The listing builds one solid part. Answer for the finished solid, in the listing's coordinates (mm). Coordinates: 2 decimals unless noted, no trailing zeros. Loops run counter-clockwise (first coordinate to the right, second up) from the corner with the lowest first, then second, coordinate; pieces in that order, holes last. Notation, with made-up numbers: M 45,67 L 97,67 A17 cw 97,80 Z; hole C -1,77 d4. An arc over 180 degrees is marked long. Return JSON: item names as keys, results as strings. Group by question number.
1. Section C-C (y = 0.8) is taken. Write down the section's boundary in (x, z) (3 decimals).
2. Given P1, Ø3, axis at x = 7.5, z = -37.5, coming from the -Y side; P2, Ø1, axis at y = 1, z = -23.5, coming from the +X side; P3, Ø1, axis at x = 12.5, y = 1.5, coming from the +Z side; P4, Ø1.6, axis at y = 2.5, z = 4.5, coming from the +X side, each flat-ended and moving along its own axis, determine where each tip first touches the part or whether it passes through.
3. Section B-B (x = 22.5) is taken. Write down the section's boundary in (y, z) (3 decimals), then the cut area to 3 significant figures.
4. Section D-D (x = 7) is taken. Write down the section's boundary in (y, z) (3 decimals).
5. Straight lines are drawn through the part: L1, parallel to X at y = 1.9, z = -5; L2, parallel to Z at x = 36, y = 1.8; L3, parallel to X at y = 1.55, z = 3.5. For each, find the intervals that lie inside material, in ascending order. Write a range as from..to.
6. Section A-A (z = -5) is taken. Write down the section's boundary in (x, y) (3 decimals).
```python
from build123d import *

# Parameters (mm, degrees)
SKETCH1_R           = 1.27
BOSS_EXTRUDE1_DEPTH = 3.175
FILLET1_R           = 2.921
SKETCH5_W           = 22
SKETCH5_H           = 3.175
BOSS_EXTRUDE3_DEPTH = 3.175
SKETCH2_W           = 6
SKETCH2_H           = 3.175
BOSS_EXTRUDE2_DEPTH = 3.175


with BuildPart() as part:
    # Sketch1 → Boss-Extrude1 (new body)
    with BuildSketch(Plane(origin=(0, 0, 0), x_dir=(1, 0, 0), z_dir=(0, 1, 0))):
        Polygon((0, 0), (0, 47.63), (10, 47.63), (39.73, 10), (39.73, 0), align=None)
        with Locations(Location((3.683, 43.74, 0), (0, 0, 270))):
            Circle(SKETCH1_R, mode=Mode.SUBTRACT)
        with Locations(Location((36.043, 5, 0), (0, 0, 270))):
            Circle(SKETCH1_R, mode=Mode.SUBTRACT)
        Polygon((10, 35.531824847), (10, 10), (30.171702171, 10), align=None, mode=Mode.SUBTRACT)
    extrude(amount=BOSS_EXTRUDE1_DEPTH)

    # Fillet1
    fillet1_edges = [part.edges().sort_by_distance(p)[0] for p in [
        (10, 1.5875, -10),
        (30.171702171, 1.5875, -10),
        (10, 1.5875, -35.531824847),
        (0, 1.5875, 0),
        (0, 1.5875, -47.63),
        (10, 1.5875, -47.63),
        (39.73, 1.5875, -10),
    ]]
    fillet(fillet1_edges, radius=FILLET1_R)

    # Sketch5 → Boss-Extrude3 (add)
    with BuildSketch(Plane.XY):
        with Locations((28.73, 1.5875)):
            Rectangle(SKETCH5_W, SKETCH5_H)
    extrude(amount=BOSS_EXTRUDE3_DEPTH)

    # Sketch2 → Boss-Extrude2 (add)
    with BuildSketch(Plane.XY.offset(3.175)):
        with Locations((21.73, 1.5875)):
            Rectangle(SKETCH2_W, SKETCH2_H)
        with Locations((35.73, 1.5875)):
            Rectangle(SKETCH2_W, SKETCH2_H)
    extrude(amount=BOSS_EXTRUDE2_DEPTH)


solid = part.part
```
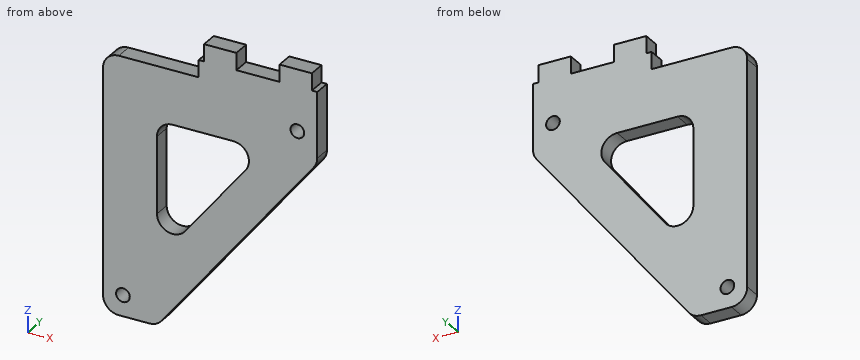
Worked out:
{
 "1": {"outline": "M 0,-44.709 A2.921 ccw 2.921,-47.63 L 8.585,-47.63 A2.921 ccw 10.877,-46.52 L 39.101,-10.796 A2.921 ccw 39.73,-8.985 L 39.73,3.175 L 38.73,3.175 L 38.73,6.35 L 32.73,6.35 L 32.73,3.175 L 24.73,3.175 L 24.73,6.35 L 18.73,6.35 L 18.73,3.175 L 17.73,3.175 L 17.73,0 L 2.921,0 A2.921 ccw 0,-2.921 Z; hole C 3.683,-43.74 d2.54; hole M 10,-27.123 A2.921 ccw 15.213,-28.934 L 26.433,-14.732 A2.921 ccw 24.141,-10 L 12.921,-10 A2.921 ccw 10,-12.921 Z; hole C 36.043,-5 d2.54"},
 "2": {"P1": "y = 0", "P2": "x = 29.46", "P3": "z = 0", "P4": "x = 38.73"},
 "3": {"outline": "M 0,-31.808 L 3.175,-31.808 L 3.175,-19.71 L 0,-19.71 Z; M 0,-10 L 3.175,-10 L 3.175,6.35 L 0,6.35 Z", "area": "90.3 mm^2"},
 "4": {"outline": "M 0,-47.63 L 3.175,-47.63 L 3.175,0 L 0,0 Z"},
 "5": {"L1": "0..34.77, 37.31..39.73", "L2": "-14.72..-6.27, -3.73..6.35", "L3": "18.73..24.73, 32.73..38.73"},
 "6": {"outline": "M 0,0 L 34.773,0 L 34.773,3.175 L 0,3.175 Z; M 37.313,0 L 39.73,0 L 39.73,3.175 L 37.313,3.175 Z"}
}
